```python
from build123d import *

# Parameters (mm, degrees)
SKETCH7_W           = 800
SKETCH7_H           = 350
BOSS_EXTRUDE1_DEPTH = 360
CUT_EXTRUDE1_DEPTH  = 642.950153828
SKETCH10_W          = 150
SKETCH10_H          = 50
CUT_EXTRUDE3_DEPTH  = 642.950153828
SKETCH11_W          = 310
SKETCH11_H          = 350
BOSS_EXTRUDE2_DEPTH = 300
SHELL3_T            = -2
SKETCH12_R          = 3
CUT_EXTRUDE4_DEPTH  = 862.452262171


with BuildPart() as part:
    # Sketch7 → Boss-Extrude1 (new body)
    with BuildSketch(Plane.XY):
        Rectangle(SKETCH7_W, SKETCH7_H)
    extrude(amount=BOSS_EXTRUDE1_DEPTH)

    # Sketch8 → Cut-Extrude1 (cut, through all)
    with BuildSketch(Plane.XZ.offset(175)):
        Polygon((-400, 280), (400, 0), (-400, 0), align=None)
    extrude(amount=-CUT_EXTRUDE1_DEPTH, mode=Mode.SUBTRACT)

    # Sketch10 → Cut-Extrude3 (cut, through all)
    with BuildSketch(Plane.XZ.offset(175)):
        with Locations((325, 335)):
            Rectangle(SKETCH10_W, SKETCH10_H)
    extrude(amount=-CUT_EXTRUDE3_DEPTH, mode=Mode.SUBTRACT)

    # Sketch11 → Boss-Extrude2 (add)
    with BuildSketch(Plane(origin=(400, 0, 0), x_dir=(0, 0, -1), z_dir=(1, 0, 0))):
        with Locations((-155, 0)):
            Rectangle(SKETCH11_W, SKETCH11_H)
    extrude(amount=BOSS_EXTRUDE2_DEPTH)

    # Shell3
    shell3_openings = [part.faces().sort_by_distance(p)[0] for p in [
        (-75, 0, 360),
        (475, 0, 310),
        (250, 0, 335),
    ]]
    offset(amount=SHELL3_T, openings=shell3_openings, kind=Kind.INTERSECTION)

    # Sketch12 → Cut-Extrude4 (cut, through all)
    with BuildSketch(Plane.XZ.offset(175)):
        with Locations(Location((-300, 345, 0), (0, 0, 270))):
            Circle(SKETCH12_R)
        with Locations(Location((-60, 345, 0), (0, 0, 270))):
            Circle(SKETCH12_R)
        with Locations(Location((180, 345, 0), (0, 0, 270))):
            Circle(SKETCH12_R)
    extrude(amount=-CUT_EXTRUDE4_DEPTH, mode=Mode.SUBTRACT)


solid = part.part
```
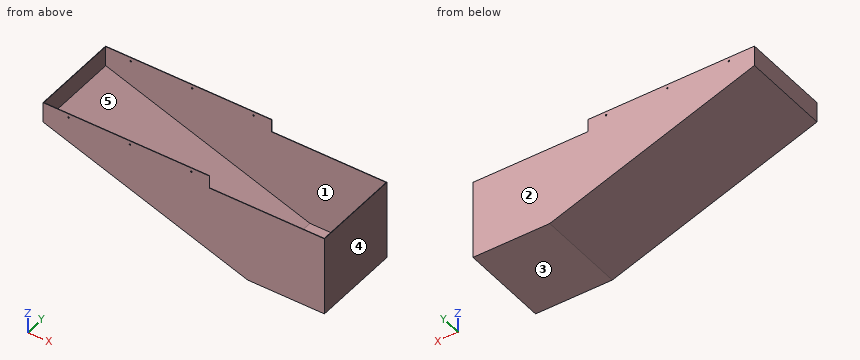
Verification items for the finished model (mm, model axes). Face numbers are marked on the shaded views. A direction names the side the tool comes from. Coordinates: 2 decimals unless noted, no trailing zeros. Write each loop counter-clockwise with the first axis right and the second up, starting at its lowest first coordinate (ties: lowest second). Pieces come first, ordered by that corner, then holes. Notation, with made-up numbers: (60.25, 88) - (71.25, 88) arc R26 cw to (71.25, 110) - close; hole circle Ø5 at (-9.5, 69). An arc over 180 degrees is marked (long way). One line per question, with ' | ' between items. Start each with the question number.
1. Gauge pin test, flat ends, axial feed: P1, Ø0.6, axis at y = 174, z = 333, coming from the +X side; P2, Ø1.5, axis at x = -223, y = -37.5, coming from the -Z side; P3, Ø12, axis at x = 47.5, y = -45.5, coming from the -Z side (3 decimals). Record the tip position at first contact, or that the pin passes through.
2. Material ranges on line 1 along X through (y, z) = (173.6, 345); line 2 along Y through (x, z) = (52.5, 311); line 3 along Z through (x, y) = (540.5, -153), recorded low to high.
3. Access from +Z, -Z, +X, -X, +Y, -Y to the whole of each face (thin tool, end or side, straight path). Record for the marked faces 4 and 5.
4. Draft check along Y on the marked faces 1, 2 and 3. Enter one of: released by +Y, released by -Y, zero draft, split by the parting line, or undercut.
5. Section check C-C (z = 177.5). Enter the section's corners in (x, y), plus the area to 3 significant figures.
6. Section check D-D (y = -115). Enter the section's corners in (x, z).
7. Section check A-A (z = 323.5). Enter the section's corners in (x, y), plus the area to 3 significant figures.
8. Section check B-B (x = 567). Enter the section's corners in (y, z).
Computed values:
1) P1: x = 250 | P2: z = 217.79 | P3: z = 121.275
2) line 1: -400 to -303, -297 to -63, -57 to 177, 183 to 250 | line 2: -175 to -173, 173 to 175 | line 3: 0 to 2
3) face 4: +Z, -Z, +X, +Y, -Y | face 5: +Z
4) face 1: undercut | face 2: released by +Y | face 3: zero draft
5) outline: (-107.14, -175) - (700, -175) - (700, 175) - (-107.14, 175) - close; hole (-101.09, -173) - (698, -173) - (698, 173) - (-101.09, 173) - close | area: 6,020 mm²
6) outline: (-400, 280) - (400, 0) - (700, 0) - (700, 310) - (698, 310) - (698, 2) - (400.34, 2) - (-398, 281.42) - (-398, 360) - (-400, 360) - close
7) outline: (-400, -175) - (250, -175) - (250, -173) - (-398, -173) - (-398, 173) - (250, 173) - (250, 175) - (-400, 175) - close | area: 3,290 mm²
8) outline: (-175, 0) - (175, 0) - (175, 310) - (173, 310) - (173, 2) - (-173, 2) - (-173, 310) - (-175, 310) - close
